Source: three-view drawing plus pictorial views. Frame: mm from the lowest corner of the part. A direction names the side the tool comes from. Give positions to 0.01 mm unless a question says otherwise; leave off trailing zeros. Order: outer loops, then holes, each group sorted by start corner. A loop starts at its lowest first (then second) coordinate and runs counter-clockwise, first axis right, second up.
1) Section B-B, the plane x = 50. Return loops of the section in (y, z).
2) Access query for the marked faces 4 and 5. Directions: +Z, -Z, +X, -X, +Y, -Y. A direction counts if a zero-diameter tool reaches every point of the face in a straight line with its end or side. Return the directions, or none.
3) Draft query along Z for the marked faces 1, 2 and 3. Return one class per face: released by +Z, released by -Z, zero draft, split by the parting line, or undercut.
4) Material intervals for line 1 (X direction, y = 4, z = 14.5); line 2 (X direction, y = 2.5, z = 103.5); line 3 (X direction, y = 24.5, z = 58), sorted ascending.
5) Section D-D, the plane y = 24.5. Return loops of the section in (x, z).
6) Section A-A, the plane y = 4.25. Return loops of the section in (x, z), plus the area to 3 significant figures.
7) Section C-C, the plane z = 108. Return loops of the section in (x, y).
8) First-contact query: P1, Ø12, axis at x = 45, z = 81.5, coming from the +Y side. Flat tip, straight axial feed; report the tip coordinate or a pass-through.
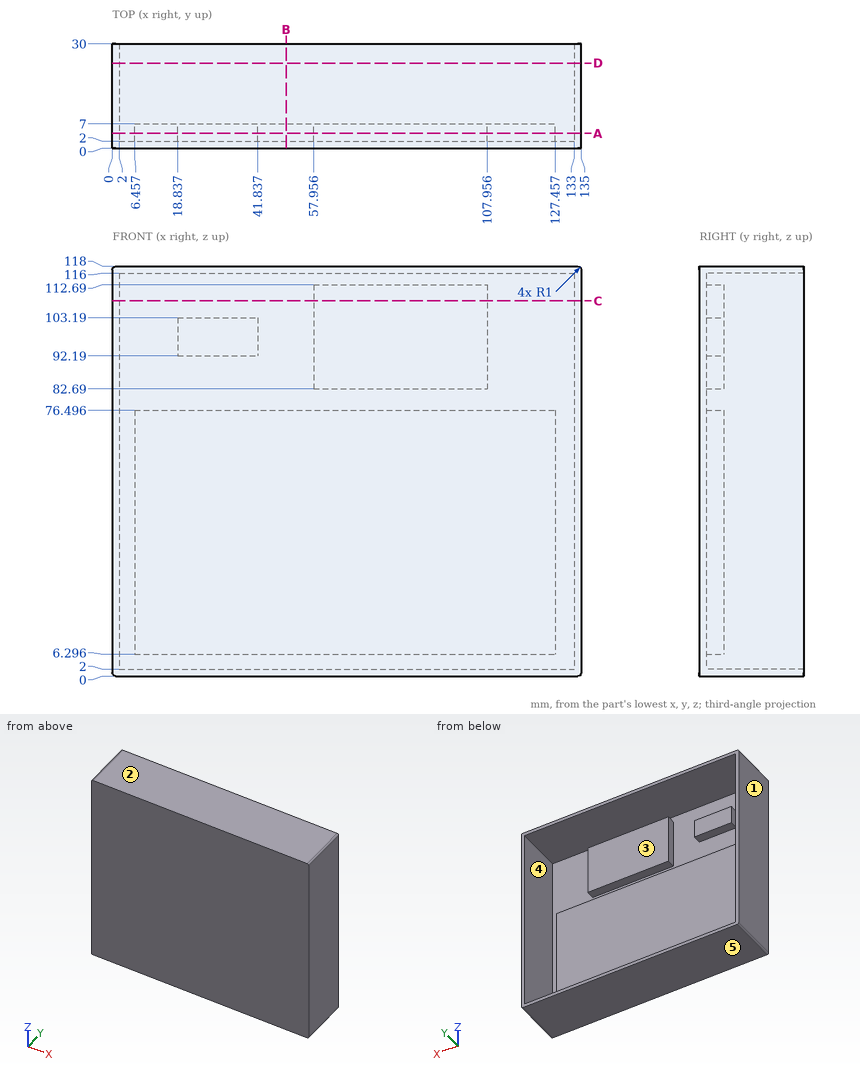
From the geometry:
1. outline: (0, 0) - (30, 0) - (30, 2) - (2, 2) - (2, 6.3) - (7, 6.3) - (7, 76.5) - (2, 76.5) - (2, 116) - (30, 116) - (30, 118) - (0, 118) - close
2. face 4: +Y
2. face 5: -Z, +X, -X, +Y, -Y
3. face 1: zero draft
3. face 2: released by +Z
3. face 3: undercut
4. line 1: x = 0 to 2, 6.46 to 127.46, 133 to 135
4. line 2: x = 0 to 2, 57.96 to 107.96, 133 to 135
4. line 3: x = 0 to 2, 133 to 135
5. outline: (0, 1) arc R1 ccw to (1, 0) - (134, 0) arc R1 ccw to (135, 1) - (135, 117) arc R1 ccw to (134, 118) - (1, 118) arc R1 ccw to (0, 117) - close; hole (2, 2) - (133, 2) - (133, 116) - (2, 116) - close
6. outline: (0, 1) arc R1 ccw to (1, 0) - (134, 0) arc R1 ccw to (135, 1) - (135, 117) arc R1 ccw to (134, 118) - (1, 118) arc R1 ccw to (0, 117) - close; (6.46, 6.3) - (127.46, 6.3) - (127.46, 76.5) - (6.46, 76.5) - close; (18.84, 92.19) - (41.84, 92.19) - (41.84, 103.19) - (18.84, 103.19) - close; (57.96, 82.69) - (107.96, 82.69) - (107.96, 112.69) - (57.96, 112.69) - close; hole (2, 2) - (133, 2) - (133, 116) - (2, 116) - close
6. area: 11,200 mm2
7. outline: (0, 0) - (135, 0) - (135, 30) - (133, 30) - (133, 2) - (107.96, 2) - (107.96, 7) - (57.96, 7) - (57.96, 2) - (2, 2) - (2, 30) - (0, 30) - close
8. P1: stops at y = 7
